Part model, mm, in its own coordinate system. Face numbers are marked on the shaded views. A direction names the side the tool comes from. Round coordinates to 2 decimals unless told otherwise and drop trailing zeros. Loops run counter-clockwise (first coordinate to the right, second up) from the corner with the lowest first, then second, coordinate; pieces in that order, holes last. Notation, with made-up numbers: (68, -3) -> (90, -3) arc R12 ccw to (90, 12) -> close; hole circle Ø7 at (52.25, 59.5). An arc over 180 degrees is marked (long way). Answer as a JSON object with one key per item and string values. Group by question number.
Autodesk Inventor part; units mm, degrees
ref_plane "YZ Plane" through (0, 0, 0) normal (1, 0, 0) x (0, 1, 0)
ref_plane "XZ Plane" through (0, 0, 0) normal (0, 1, 0) x (-1, 0, 0)
ref_plane "XY Plane" through (0, 0, 0) normal (0, 0, 1) x (1, 0, 0)
sketch "Эскиз1" plane through (0, 0, 0) normal (0, 1, 0) x (-1, 0, 0)
  circle A0 centre (0, 0) radius 2.7
  circle A1 centre (0, 0) radius 4
  dimension "d13" = 5.4
  dimension "d14" = 8
extrude "Выдавливание1" add sketch "Эскиз1" along normal blind 9.5
sketch "Эскиз2" plane through (0, 9.5, 0) normal (0, 1, 0) x (1, 0, 0)
  circle A0 centre (0, 0) radius 1.6
  circle A1 centre (0, 0) radius 6
  circle A2 centre (0, 0) radius 2.7
  dimension "d15" = 12
extrude "Выдавливание2" add sketch "Эскиз2" against normal blind 2 contours A1
sketch "Эскиз3" plane through (0, 0, 0) normal (0, -1, 0) x (1, 0, 0)
  circle A0 centre (0, 0) radius 2.7
  circle A1 centre (0, 0) radius 6
extrude "Выдавливание3" add sketch "Эскиз3" against normal blind 2
sketch "Эскиз4" plane through (0, 0, 0) normal (0, 0, 1) x (1, 0, 0)
  line L0 (-2.7, 9.5) -> (2.7, 9.5)
  line L1 (0, 9.5) -> (0, 0)
  line L2 (6, 9.5) -> (6, 7.5)
  line L3 (-4, 7.5) -> (4, 7.5)
  line L4 (6, 8.5) -> (4, 7.5)
  line L5 (6, 8.5) -> (6, 7.5)
  line L6 (-6, 7.5) -> (6, 7.5)
  line L7 (4, 7.5) -> (6, 7.5)
  line L8 (6, 0) -> (6, 2)
  line L9 (6, 1) -> (4, 2)
  line L10 (4, 2) -> (6, 2)
  line L11 (6, 1) -> (6, 2)
  point P0 (5.5, 0)
revolve "Вращение1" cut sketch "Эскиз4" angle 360 about axis through (0, 9.5, 0) along (0, -1, 0)
fillet "Сопряжение1" radius 1 4 edges at (0, 7.5, -4) (0, 7.5, 4) (0, 2, -4) (0, 2, 4)
fillet "Сопряжение2" radius 0.7 2 edges at (2.7, 0, 0) (2.7, 9.5, 0)
properties part number "rolik"
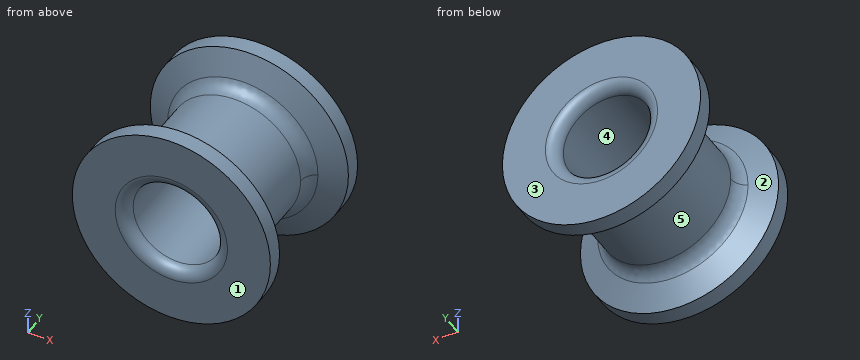
Item 1: Drop flat-ended pins along their axis: pin 1 Ø1.5 at (x, y) = (1.5, 8) entering from -Z; pin 2 Ø1 at (x, y) = (-1.5, 3.5) entering from +Z; pin 3 Ø3 at (y, z) = (7.5, 2.5) entering from +X. Give the stop position or say it passes through.
Item 2: Band-saw the part on A-A, the plane y = 5.5. List the corners of the cut face in (x, z).
Item 3: Which spindle directions (+Z, -Z, +X, -X, +Y, -Y) get a long thin tool onto all of the face, cutting with end or side? Do the marked faces 1 and 2. Say none if no direction does.
Item 4: Drill centre lines: line 1 (Z direction, x = 0, y = 5.5); line 2 (X direction, y = 8.75, z = 1.5) (3 decimals); line 3 (Y direction, x = 3, z = -3.75). Where is each one in solid material? Low to high.
Item 5: Two-plate mould, pull along X, no slides. Class the marked faces 3, 4 and 5: pulls with the +X half, pulls with the -X half, needs draft (parallel to the pull), parting line crosses it, or undercut.
Entries:
{
 "1": {"pin 1": "z = -5.93", "pin 2": "z = 3.87", "pin 3": "x = 5.84"},
 "2": {"outline": "circle Ø8 at (0, 0); hole circle Ø5.4 at (0, 0)"},
 "3": {"face 1": "+Z, -Z, +X, -X, -Y", "face 2": "none"},
 "4": {"line 1": "-4 to -2.7, 2.7 to 4", "line 2": "-5.809 to -2.245, 2.245 to 5.809", "line 3": "0 to 1.6, 7.9 to 9.5"},
 "5": {"face 3": "needs draft", "face 4": "undercut", "face 5": "parting line crosses it"}
}
